Work out the finished part from the listing and answer in its coordinate system (mm). A direction names the side the tool comes from. Round coordinates to 2 decimals unless told otherwise and drop trailing zeros. Answer as a JSON object with one key per item and string values.
```python
from build123d import *

# Parameters (mm, degrees)
SKETCH1_W                                           = 85
SKETCH1_H                                           = 210
BOSS_EXTRUDE1_DEPTH                                 = 10
CBORE_FOR_4_BINDING_HEAD_MACHINE_SCREW1_D           = 3.4544
CBORE_FOR_4_BINDING_HEAD_MACHINE_SCREW1_CBORE_D     = 6.74624
CBORE_FOR_4_BINDING_HEAD_MACHINE_SCREW1_CBORE_DEPTH = 1.7272
CBORE_FOR_4_BINDING_HEAD_MACHINE_SCREW2_D           = 3.2639
CBORE_FOR_4_BINDING_HEAD_MACHINE_SCREW2_DEPTH       = 10
CBORE_FOR_4_BINDING_HEAD_MACHINE_SCREW2_CBORE_D     = 6.74624
CBORE_FOR_4_BINDING_HEAD_MACHINE_SCREW2_CBORE_DEPTH = 1.7272
SKETCH10_R                                          = 6.35
SKETCH10_R_2                                        = 4.5
CUT_EXTRUDE1_DEPTH                                  = 5
CUT_EXTRUDE3_REACH                                  = 12
SKETCH10_3_R                                        = 4.5
F_4_40_TAPPED_HOLE2_D                               = 2.2606
F_4_40_TAPPED_HOLE2_DEPTH                           = 7.6
F_4_40_TAPPED_HOLE2_TIP                             = 0.679152758


with BuildPart() as part:
    # Sketch1 → Boss-Extrude1 (new body)
    with BuildSketch(Plane.XY):
        with Locations((-115.863171355, -13.158567775)):
            Rectangle(SKETCH1_W, SKETCH1_H)
    extrude(amount=BOSS_EXTRUDE1_DEPTH)

    # CBORE for #4 Binding Head Machine Screw1 (through all)
    with Locations(Plane(origin=(0, 0, 0), x_dir=(-1, 0, 0), z_dir=(0, 0, -1))):
        with Locations((78.363171355, 51.841432225), (78.363171355, -13.158567775), (78.363171355, -78.158567775)):
            CounterBoreHole(CBORE_FOR_4_BINDING_HEAD_MACHINE_SCREW1_D / 2, CBORE_FOR_4_BINDING_HEAD_MACHINE_SCREW1_CBORE_D / 2, CBORE_FOR_4_BINDING_HEAD_MACHINE_SCREW1_CBORE_DEPTH)

    # CBORE for #4 Binding Head Machine Screw2
    with Locations(Plane(origin=(0, 0, 0), x_dir=(-1, 0, 0), z_dir=(0, 0, -1))):
        with Locations((88.363171355, 86.841432225), (115.863171355, 86.841432225), (143.363171355, 86.841432225), (143.363171355, -113.158567775), (115.863171355, -113.158567775), (88.363171355, -113.158567775)):
            CounterBoreHole(CBORE_FOR_4_BINDING_HEAD_MACHINE_SCREW2_D / 2, CBORE_FOR_4_BINDING_HEAD_MACHINE_SCREW2_CBORE_D / 2, CBORE_FOR_4_BINDING_HEAD_MACHINE_SCREW2_CBORE_DEPTH, depth=CBORE_FOR_4_BINDING_HEAD_MACHINE_SCREW2_DEPTH)

    # Sketch10 → Cut-Extrude1 (cut)
    with BuildSketch(Plane(origin=(0, 0, 0), x_dir=(-1, 0, 0), z_dir=(0, 0, -1))):
        with Locations((113.363171355, -53.158567775)):
            Circle(SKETCH10_R)
        with Locations((113.363171355, -53.158567775)):
            Circle(SKETCH10_R_2, mode=Mode.SUBTRACT)
    extrude(amount=-CUT_EXTRUDE1_DEPTH, mode=Mode.SUBTRACT)

    # Sketch10<3> → Cut-Extrude3 (cut, up to next)
    with BuildSketch(Plane(origin=(0, 0, 0), x_dir=(-1, 0, 0), z_dir=(0, 0, -1)), mode=Mode.PRIVATE) as cut_extrude3_sk1:
        with Locations((113.363171355, -53.158567775)):
            Circle(SKETCH10_3_R)
    cut_extrude3_tool1 = extrude(cut_extrude3_sk1.sketch, amount=-CUT_EXTRUDE3_REACH, mode=Mode.PRIVATE) & part.part
    add(cut_extrude3_tool1.solids().sort_by_distance((-113.363171, -53.158568, 0))[0], mode=Mode.SUBTRACT)

    # #4-40 Tapped Hole2
    with Locations(Plane.ZY.offset(158.363171355)):
        with Locations((5, -63.158567775), (5, 36.841432225)):
            Hole(F_4_40_TAPPED_HOLE2_D / 2, depth=F_4_40_TAPPED_HOLE2_DEPTH)
            with Locations((0, 0, -(F_4_40_TAPPED_HOLE2_DEPTH + F_4_40_TAPPED_HOLE2_TIP / 2))):  # 118° drill point
                Cone(0, F_4_40_TAPPED_HOLE2_D / 2, F_4_40_TAPPED_HOLE2_TIP, mode=Mode.SUBTRACT)


solid = part.part
```
Item 1: Consider line 1 along Y through (x, z) = (-88, 4.75); line 2 along X through (y, z) = (-78.5, 1); line 3 along Y through (x, z) = (-114, 8.25). Determine where each line is inside the solid, lowest interval first.
Results found:
{"line 1": "-118.16 to -114.75, -111.57 to 85.25, 88.43 to 91.84", "line 2": "-158.36 to -81.72, -75.01 to -73.36", "line 3": "-118.16 to -57.61, -48.7 to 91.84"}
Item 2: For faces 4 (the flat face through (-116, -118.159, 5)), 5 (the flat face through (-116, -57, 5)), determine the directions among +Z, -Z, +X, -X, +Y, -Y from which every point of the face is accessible in a straight line to the end or side of a thin tool.
Results found:
{"face 4": "+Z, -Z, +X, -X, -Y", "face 5": "-Z"}
Item 3: Determine the mould class of faces 1 (the flat face through (-116, 91.841, 5)), 2 (the flat face through (-80, -15, 1.727)), 3 (the flat face through (-73.363, -15, 5)) for opening direction Y: pulls with the +Y half, pulls with the -Y half, needs draft (parallel to the pull), parting line crosses it, or undercut.
Results found:
{"face 1": "pulls with the +Y half", "face 2": "undercut", "face 3": "needs draft"}
Item 4: This flat-tipped pin is pushed along its axis until it touches: P1, Ø5.5, axis at x = -78.36, y = -78.16, coming from the -Z side. Where does it stop, or does it pass through?
Results found:
{"P1": "z = 1.73"}
